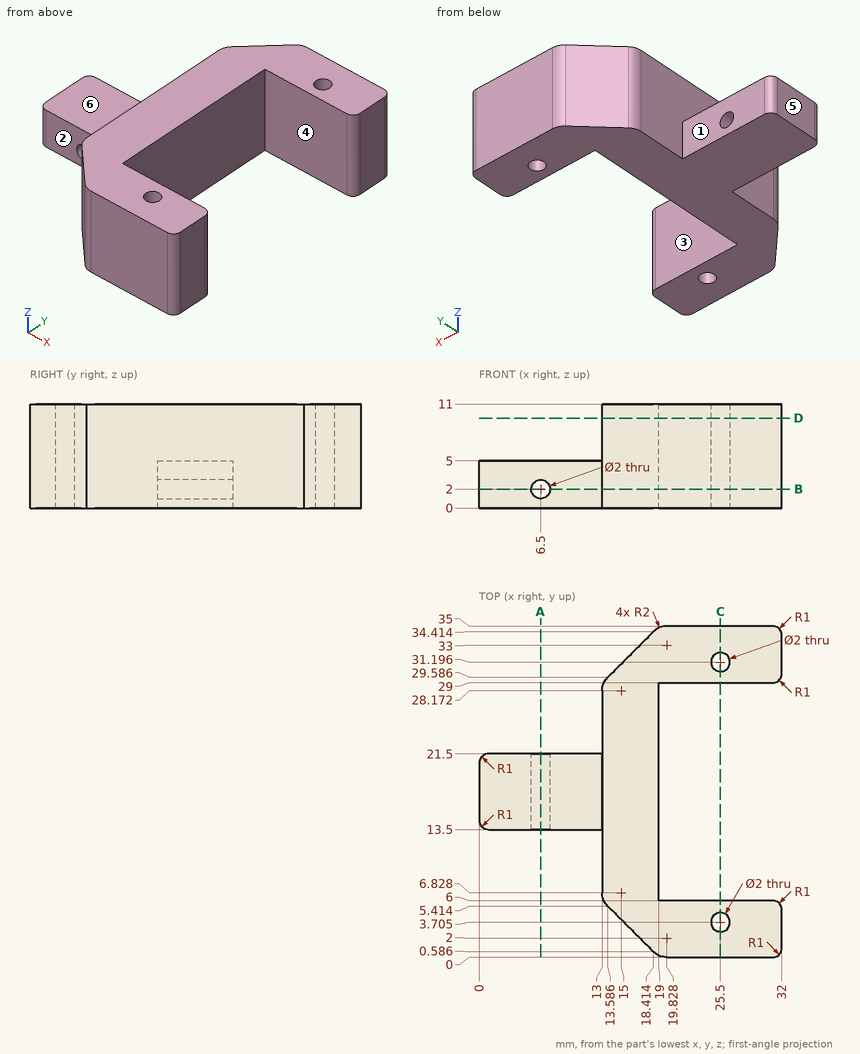
Input: dimensioned drawing with shaded views. Units: mm. Origin: part minimum x, y, z. A direction names the side the tool comes from. Give positions to 0.01 mm unless a question says otherwise; leave off trailing zeros. Loops run counter-clockwise (first coordinate to the right, second up) from the corner with the lowest first, then second, coordinate; pieces in that order, holes last. Notation, with made-up numbers: (46.25, 9.5) -> (94.25, 9.5) arc R21 ccw to (94.25, 28.5) -> close; hole circle Ø7 at (52.25, -4.75). An arc over 180 degrees is marked (long way). Use a Markdown table: item, result.
Q1. Section query D-D, the plane z = 9.5. Return the cut outline in (x, y) (1 decimal).
Entries:
| item | result |
|---|---|
| outline | (13, 6.8) arc R2 ccw to (13.6, 5.4) -> (18.4, 0.6) arc R2 ccw to (19.8, 0) -> (31, 0) arc R1 ccw to (32, 1) -> (32, 5) arc R1 ccw to (31, 6) -> (19, 6) -> (19, 29) -> (31, 29) arc R1 ccw to (32, 30) -> (32, 34) arc R1 ccw to (31, 35) -> (19.8, 35) arc R2 ccw to (18.4, 34.4) -> (13.6, 29.6) arc R2 ccw to (13, 28.2) -> close; hole circle Ø2 at (25.5, 3.7); hole circle Ø2 at (25.5, 31.2) |
Q2. Ray query, probe 1 along Y at (x, z) = (25.5, 5.25) (1 decimal); probe 2 along X at (y, z) = (19, 2); probe 3 along Y at (x, z) = (23.5, 2.75). Return the intervals inside material, ascending. Write a range as from..to.
Entries:
| item | result |
|---|---|
| probe 1 | y = 0..2.7, 4.7..6, 29..30.2, 32.2..35 |
| probe 2 | x = 0..5.5, 7.5..19 |
| probe 3 | y = 0..6, 29..35 |
Q3. Section query B-B, the plane z = 2. State how many separate pieces and enclosed holes the cut face has, plus the area to 3 significant figures.
Entries:
| item | result |
|---|---|
| separate pieces | 2 |
| enclosed holes | 2 |
| area | 410 mm² |
Q4. Section query A-A, the plane x = 6.5. Return the cut outline in (y, z).
Entries:
| item | result |
|---|---|
| outline | (13.5, 0) -> (21.5, 0) -> (21.5, 1) -> (13.5, 1) -> close; (13.5, 3) -> (21.5, 3) -> (21.5, 5) -> (13.5, 5) -> close |
Q5. Section query C-C, the plane x = 25.5. Return the cut outline in (y, z) (1 decimal).
Entries:
| item | result |
|---|---|
| outline | (0, 0) -> (2.7, 0) -> (2.7, 11) -> (0, 11) -> close; (4.7, 0) -> (6, 0) -> (6, 11) -> (4.7, 11) -> close; (29, 0) -> (30.2, 0) -> (30.2, 11) -> (29, 11) -> close; (32.2, 0) -> (35, 0) -> (35, 11) -> (32.2, 11) -> close |
Q6. Pull-direction query (Y, two-part tool) for the marked faces 1, 2 and 3; classes: pulls with the +Y half, pulls with the -Y half, needs draft (parallel to the pull), parting line crosses it, or undercut.
Entries:
| item | result |
|---|---|
| face 1 | pulls with the +Y half |
| face 2 | pulls with the -Y half |
| face 3 | undercut |
Q7. Access query for the marked faces 4, 5 and 6. Directions: +Z, -Z, +X, -X, +Y, -Y. A direction counts if a zero-diameter tool reaches every point of the face in a straight line with its end or side. Return the directions, or none.
Entries:
| item | result |
|---|---|
| face 4 | +Z, -Z, +X |
| face 5 | +Z, -Z, -X, +Y, -Y |
| face 6 | +Z, -X, +Y, -Y |
Q8. First-contact query: P1, Ø4, axis at x = 9, z = 2.5, coming from the +Y side; P2, Ø5.5, axis at x = 9.5, z = 3.5, coming from the -Y side; P3, Ø5.5, axis at y = 13, z = 4, coming from the +X side; P4, Ø1.8, axis at x = 25.5, y = 3.7, coming from the -Z side. Flat tips, straight axial feed; report the tip coordinate or a pass-through.
Entries:
| item | result |
|---|---|
| P1 | stops at y = 21.5 |
| P2 | stops at y = 13.5 |
| P3 | stops at x = 19 |
| P4 | passes through |
